Study the drawing (mm; zero at the part's minimum x, y, z) and answer. A direction names the side the tool comes from. Coordinates: 2 decimals unless noted, no trailing zeros. Loops run counter-clockwise (first coordinate to the right, second up) from the corner with the lowest first, then second, coordinate; pieces in that order, holes last.
Q1. Section A-A (y = 6.5) is taken. Give the vertices of the cut face in (x, z) (1 decimal).
Q2. Which of the six approach directions +Z, -Z, +X, -X, +Y, -Y give full straight-line access (tool end or side, diameter ignored) to the marked faces 4 and 5?
Q3. Straight lines are drawn through the part: line 1 (Y direction, x = 6.5, z = 3.15); line 2 (Y direction, x = 4.5, z = 3.95) (1 decimal); line 3 (X direction, y = 5.75, z = 4.05). For each, find the intervals that lie inside material, in ascending order.
Q4. The mould has two halves that part along X. Classify the marked faces 1, 2 and 3: pulls with the +X half, pulls with the -X half, needs draft (parallel to the pull), parting line crosses it, or undercut.
Q5. Section D-D (x = 1) is taken. Give the vertices of the cut face in (y, z) (1 decimal), then the cut area to 3 significant figures.
Q6. Section C-C (z = 4.95) is taken. Give the vertices of the cut face in (x, y).
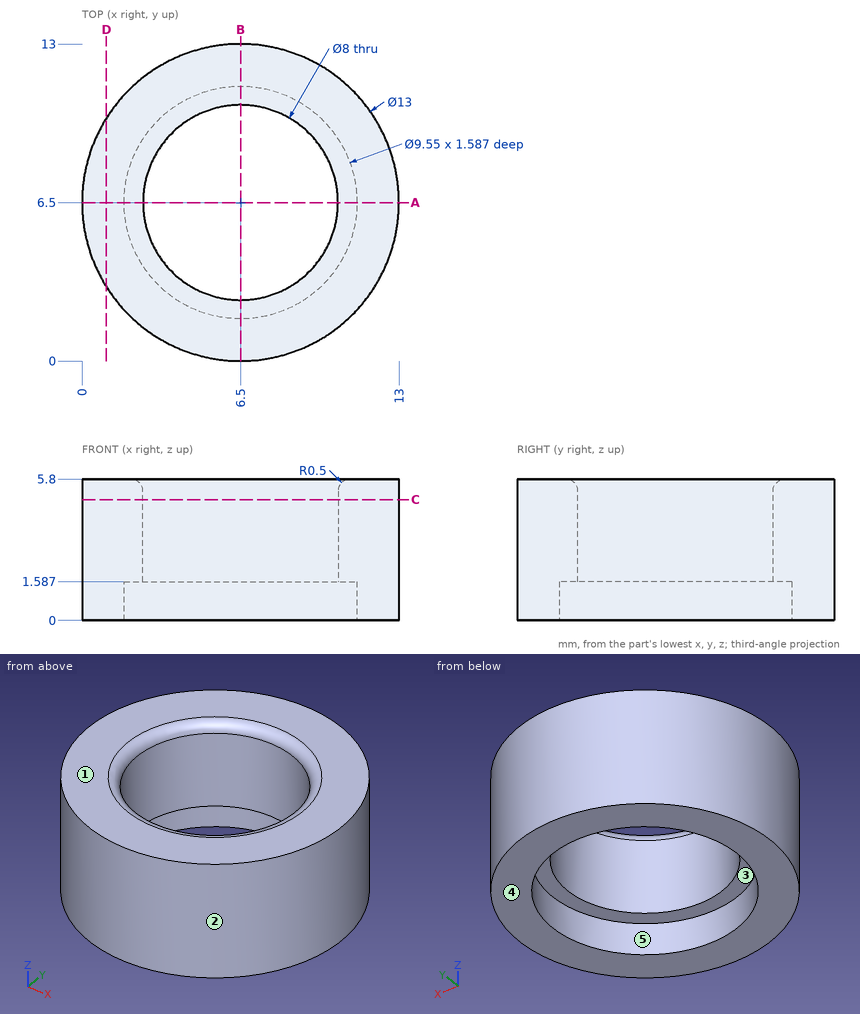
Numbers:
1. outline: (0, 0) - (1.7, 0) - (1.7, 1.6) - (2.5, 1.6) - (2.5, 5.3) arc R0.5 ccw to (2, 5.8) - (0, 5.8) - close; (10.5, 1.6) - (11.3, 1.6) - (11.3, 0) - (13, 0) - (13, 5.8) - (11, 5.8) arc R0.5 ccw to (10.5, 5.3) - close
2. face 4: -Z, +X, -X, +Y, -Y
2. face 5: -Z
3. line 1: y = 0 to 2.5, 10.5 to 13
3. line 2: y = 0.3 to 3, 10 to 12.7
3. line 3: x = 0.04 to 2.57, 10.43 to 12.96
4. face 1: needs draft
4. face 2: parting line crosses it
4. face 3: undercut
5. outline: (3, 0) - (10, 0) - (10, 5.8) - (3, 5.8) - close
5. area: 40.2 mm2
6. outline: circle Ø13 at (6.5, 6.5); hole circle Ø8 at (6.5, 6.5)
